Here's how the part is built. I have some questions about the finished solid (model axes, mm). A direction names the side the tool comes from. Coordinates: 2 decimals unless noted, no trailing zeros. Order: outer loops, then holes, each group sorted by start corner. A loop starts at its lowest first (then second) coordinate and runs counter-clockwise, first axis right, second up. Notation, with made-up numbers: M 86,42 L 130,42 A20 cw 130,55 Z; hole C 35,29 d4. An arc over 180 degrees is marked long. Answer as CSV lines item,"result". Start each with the question number.
```python
from build123d import *

# Parameters (mm, degrees)
SKETCH1_W                = 80
SKETCH1_H                = 60
BOSS_EXTRUDE1_DEPTH      = 60
SKETCH2_W                = 95.889864734
SKETCH2_H                = 40
CUT_EXTRUDE1_DEPTH       = 50
SKETCH3_W                = 80
SKETCH3_H                = 10
CUT_EXTRUDE2_DEPTH       = 30
SKETCH5_R                = 4.1
CUT_EXTRUDE3_DEPTH       = 7
SKETCH8_R                = 10.75
CUT_EXTRUDE5_DEPTH       = 88.749643874
SKETCH12_R               = 2.05
CUT_EXTRUDE8_DEPTH       = 88.749643874
FILLET1_R                = 2
SKETCH13_R               = 2.55
CUT_EXTRUDE9_DEPTH       = 88.749643874
SKETCH6_W                = 7
SKETCH6_H                = 16.599779926
BOSS_EXTRUDE2_DEPTH      = 20
CUT_EXTRUDE10_DEPTH      = 97.953597148
CUT_EXTRUDE10_DEPTH_BACK = 97.953597148
BOSS_EXTRUDE3_DEPTH      = 40


with BuildPart() as part:
    # Sketch1 → Boss-Extrude1 (new body)
    with BuildSketch(Plane(origin=(0, 0, 0), x_dir=(1, 0, 0), z_dir=(0, 1, 0))):
        Rectangle(SKETCH1_W, SKETCH1_H)
    extrude(amount=BOSS_EXTRUDE1_DEPTH)

    # Sketch2 → Cut-Extrude1 (cut)
    with BuildSketch(Plane(origin=(0, 60, 0), x_dir=(1, 0, 0), z_dir=(0, 1, 0))):
        Rectangle(SKETCH2_W, SKETCH2_H)
    extrude(amount=-CUT_EXTRUDE1_DEPTH, mode=Mode.SUBTRACT)

    # Sketch3 → Cut-Extrude2 (cut)
    with BuildSketch(Plane(origin=(0, 60, 0), x_dir=(1, 0, 0), z_dir=(0, 1, 0))):
        with Locations((0, -25)):
            Rectangle(SKETCH3_W, SKETCH3_H)
    extrude(amount=-CUT_EXTRUDE2_DEPTH, mode=Mode.SUBTRACT)

    # Sketch5 → Cut-Extrude3 (cut)
    with BuildSketch(Plane.XZ):
        with Locations(Location((-30, 0.5, 0), (0, 0, 270))):
            Circle(SKETCH5_R)
        with Locations(Location((30, 0.5, 0), (0, 0, 90))):
            Circle(SKETCH5_R)
    extrude(amount=-CUT_EXTRUDE3_DEPTH, mode=Mode.SUBTRACT)

    # Sketch8 → Cut-Extrude5 (cut, through all)
    with BuildSketch(Plane.XY.offset(-20)):
        with Locations((0, 35)):
            Circle(SKETCH8_R)
    extrude(amount=-CUT_EXTRUDE5_DEPTH, mode=Mode.SUBTRACT)

    # Sketch12 → Cut-Extrude8 (cut, through all)
    with BuildSketch(Plane.XY.offset(-20)):
        with Locations((15.5, 50.5)):
            Circle(SKETCH12_R)
        with Locations((-15.5, 19.5)):
            Circle(SKETCH12_R)
        with Locations((-15.5, 50.5)):
            Circle(SKETCH12_R)
        with Locations((15.5, 19.5)):
            Circle(SKETCH12_R)
    extrude(amount=-CUT_EXTRUDE8_DEPTH, mode=Mode.SUBTRACT)

    # Fillet1
    fillet1_edges = [part.edges().sort_by_distance(p)[0] for p in [
        (-40, 60, -25),
        (40, 60, -25),
        (-40, 30, 25),
        (0, 30, 20),
        (40, 30, 25),
        (0, 0, -30),
        (-40, 30, -30),
        (40, 30, -30),
        (0, 60, -30),
    ]]
    fillet(fillet1_edges, radius=FILLET1_R)

    # Sketch13 → Cut-Extrude9 (cut, through all)
    with BuildSketch(Plane(origin=(0, 0, 20), x_dir=(-1, 0, 0), z_dir=(0, 0, -1))):
        with Locations((-34, 19)):
            Circle(SKETCH13_R)
        with Locations((34, 19)):
            Circle(SKETCH13_R)
    extrude(amount=-CUT_EXTRUDE9_DEPTH, mode=Mode.SUBTRACT)

    # Sketch6 → Boss-Extrude2 (add)
    with BuildSketch(Plane(origin=(0, 0, 20), x_dir=(-1, 0, 0), z_dir=(0, 0, -1))):
        with Locations((-26.5, 18.299889963)):
            Rectangle(SKETCH6_W, SKETCH6_H)
        with Locations((26.5, 18.299889963)):
            Rectangle(SKETCH6_W, SKETCH6_H)
    extrude(amount=BOSS_EXTRUDE2_DEPTH)

    # Sketch14 → Cut-Extrude10 (cut, two sides: drawn at the far end of the back side and taken through both)
    with BuildSketch(Plane.ZY.offset(30).offset(-CUT_EXTRUDE10_DEPTH_BACK)):
        Polygon((0, 10), (20, 26.599779926), (0, 26.599779926), align=None)
    extrude(amount=CUT_EXTRUDE10_DEPTH + CUT_EXTRUDE10_DEPTH_BACK, mode=Mode.SUBTRACT)

    # Sketch15 → Boss-Extrude3 (add, symmetric)
    with BuildSketch(Plane(origin=(0, 0, 0), x_dir=(0, 0, -1), z_dir=(1, 0, 0))):
        Polygon((20, 13.27), (16.846771097, 10), (20, 10), align=None)
    extrude(amount=BOSS_EXTRUDE3_DEPTH, both=True)


solid = part.part
```
1) If we mould it in two halves opening along Y, with no side actions, what happens to faces 5 (the face through (39.4, 29.43, 24.93)), 6 (the face through (-39.43, 29.41, -29.4)), 7 (the face through (36.548, 19.112, 24.93))? For each: released by +Y, released by -Y, zero draft, split by the parting line, or undercut.
2) Which directions (+Z, -Z, +X, -X, +Y, -Y) give clear straight access to the entire face, cutting with the end or side of a thin tool? Please do faces 1 (the face through (-23, 16, 12)), 2 (the face through (30, 16, 12)), 3 (the face through (0.56, 11.66, -18.45)), 4 (the face through (-30, 7, 1)).
3) Suppose I cut it at C-C on x = 0. Please give me the cut outline in (y, z).
4) Suppose I cut it at B-B on y = 50.5. Please give me the cut outline in (x, z).
5) Suppose I cut it at A-A on x = -15.5. Please give me the cut outline in (y, z).
6) Will these pins go through, and if not, where does the flat tip stop? pin 1 Ø5 at (y, z) = (20, 11.5) entering from +X; pin 2 Ø5 at (y, z) = (19, 10) entering from -X; pin 3 Ø2.5 at (x, z) = (-30, 1) entering from -Y; pin 4 Ø10 at (y, z) = (22, 6) entering from -X.
7) Suppose I cut it at D-D on z = -25. Please give me the cut outline in (x, y).
8) I need wall thicknesses on line 1 (Z direction, x = -5.5, y = 17); line 2 (X direction, y = 50, z = -22); line 3 (X direction, y = 12, z = 16). Which ranges of each line are inside material? Lowest first, please. Write a range as [from, to].
Output:
1,face 5,"released by +Y"
1,face 6,"zero draft"
1,face 7,"undercut"
2,face 1,"+Y"
2,face 2,"+X, +Y"
2,face 3,"+X, -X, +Y"
2,face 4,"-Y"
3,outline,"M 0,-28 A2 ccw 2,-30 L 24.25,-30 L 24.25,-20 L 13.27,-20 L 10,-16.85 L 10,20 L 28,20 A2 ccw 30,22 L 30,30 L 0,30 Z; M 45.75,-30 L 58,-30 A2 ccw 60,-28 L 60,-20 L 45.75,-20 Z"
4,outline,"M -40,-28 A2 ccw -38,-30 L -17.55,-30 L -17.55,-20 L -40,-20 Z; M -13.45,-30 L 13.45,-30 L 13.45,-20 L -13.45,-20 Z; M 17.55,-30 L 38,-30 A2 ccw 40,-28 L 40,-20 L 17.55,-20 Z"
5,outline,"M 0,-28 A2 ccw 2,-30 L 17.45,-30 L 17.45,-20 L 13.27,-20 L 10,-16.85 L 10,20 L 28,20 A2 ccw 30,22 L 30,30 L 0,30 Z; M 21.55,-30 L 48.45,-30 L 48.45,-20 L 21.55,-20 Z; M 52.55,-30 L 58,-30 A2 ccw 60,-28 L 60,-20 L 52.55,-20 Z"
6,pin 1,"x = 30"
6,pin 2,"x = -30"
6,pin 3,"y = 7"
6,pin 4,"through"
7,outline,"M -40,0 L 40,0 L 40,58 A2 ccw 38,60 L -38,60 A2 ccw -40,58 Z; hole C -15.5,19.5 d4.1; hole C -15.5,50.5 d4.1; hole C 0,35 d21.5; hole C 15.5,19.5 d4.1; hole C 15.5,50.5 d4.1"
8,line 1,"[-30, -20], [20, 30]"
8,line 2,"[-40, -17.49], [-13.51, 13.51], [17.49, 40]"
8,line 3,"[-30, -23], [23, 30]"
